Geometry: final body of the model. Coordinates: model frame, mm. A direction names the side the tool comes from. Give positions to 0.01 mm unless a question says otherwise; leave off trailing zeros. Order: outer loops, then holes, each group sorted by start corner. A loop starts at its lowest first (then second) coordinate and runs counter-clockwise, first axis right, second up. Notation, with made-up numbers: (-24.5, 85) - (-20.5, 85) arc R27 ccw to (-20.5, 101) - close; hole circle Ø5 at (87.25, 37.25). An arc over 180 degrees is marked (long way). One line per item, written item: value.
```python
from build123d import *

# Parameters (mm, degrees)
SKETCH_1_R          = 12.5
EXTRUDE_1_DEPTH     = 8.2
SKETCH_2_R          = 12.5
EXTRUDE_2_DEPTH     = 3
SKETCH_3_W          = 10
SKETCH_3_H          = 10
EXTRUDE_3_DEPTH     = 11.2
FILLET_1_R          = 10
SKETCH_4_R          = 2.5
CUT_EXTRUDE_4_DEPTH = 28.240939498
SKETCH_5_R          = 5.5
CUT_EXTRUDE_5_DEPTH = 4


with BuildPart() as part:
    # Эскиз1 → Вытянуть1 (new body)
    with BuildSketch(Plane(origin=(0, 0, 0), x_dir=(1, 0, 0), z_dir=(0, 1, 0))):
        with Locations(Location((0, 0, 0), (0, 0, 270))):
            Circle(SKETCH_1_R)
        Polygon((8.5, -4.907477288), (8.5, 4.907477288), (0, 9.814954576), (-8.5, 4.907477288), (-8.5, -4.907477288), (0, -9.814954576), align=None, mode=Mode.SUBTRACT)
    extrude(amount=EXTRUDE_1_DEPTH)

    # Эскиз2 → Вытянуть2 (add)
    with BuildSketch(Plane(origin=(0, 8.2, 0), x_dir=(1, 0, 0), z_dir=(0, 1, 0))):
        with Locations(Location((0, 0, 0), (0, 0, 270))):
            Circle(SKETCH_2_R)
    extrude(amount=EXTRUDE_2_DEPTH)

    # Эскиз3 → Вытянуть3 (add)
    with BuildSketch(Plane.XZ):
        with Locations((16.456439237, 0)):
            Rectangle(SKETCH_3_W, SKETCH_3_H)
        with Locations((-16.456439237, 0)):
            Rectangle(SKETCH_3_W, SKETCH_3_H)
    extrude(amount=-EXTRUDE_3_DEPTH)

    # Скругление1
    fillet_1_edges = [part.edges().sort_by_distance(p)[0] for p in [
        (11.456439237, 5.6, 5),
        (11.456439237, 5.6, -5),
        (-11.456439237, 5.6, -5),
        (-11.456439237, 5.6, 5),
    ]]
    fillet(fillet_1_edges, radius=FILLET_1_R)

    # Эскиз4 → Вытянуть4 (cut, through all)
    with BuildSketch(Plane(origin=(0, 11.2, 0), x_dir=(1, 0, 0), z_dir=(0, 1, 0))):
        with Locations(Location((16.456439237, 0, 0), (0, 0, 270))):
            Circle(SKETCH_4_R)
        with Locations(Location((-16.456439237, 0, 0), (0, 0, 270))):
            Circle(SKETCH_4_R)
    extrude(amount=-CUT_EXTRUDE_4_DEPTH, mode=Mode.SUBTRACT)

    # Эскиз5 → Вытянуть5 (cut)
    with BuildSketch(Plane(origin=(0, 11.2, 0), x_dir=(1, 0, 0), z_dir=(0, 1, 0))):
        with Locations(Location((0, 0, 0), (0, 0, 270))):
            Circle(SKETCH_5_R)
    extrude(amount=-CUT_EXTRUDE_5_DEPTH, mode=Mode.SUBTRACT)


solid = part.part
```
1) Section B-B, the plane x = 17.5. Return loops of the section in (y, z).
Answers below:
outline: (0, -5) - (11.2, -5) - (11.2, -2.27) - (0, -2.27) - close; (0, 2.27) - (11.2, 2.27) - (11.2, 5) - (0, 5) - close
2) Material intervals for line 1 along X through (y, z) = (10.5, 0); line 2 along X through (y, z) = (3.25, 0); line 3 along X through (y, z) = (1, 3), sorted ascending.
Answers below:
line 1: -21.46 to -18.96, -13.96 to -5.5, 5.5 to 13.96, 18.96 to 21.46
line 2: -21.46 to -18.96, -13.96 to -8.5, 8.5 to 13.96, 18.96 to 21.46
line 3: -21.46 to -8.5, 8.5 to 21.46
3) Section D-D, the plane z = 7.5. Return loops of the section in (x, y).
Answers below:
outline: (-10.16, 0) - (-4.01, 0) - (-4.01, 8.2) - (4.01, 8.2) - (4.01, 0) - (10.16, 0) - (10.16, 11.2) - (-10.16, 11.2) - close
4) Section A-A, the plane z = 0. Return loops of the section in (x, y).
Answers below:
outline: (-21.46, 0) - (-18.96, 0) - (-18.96, 11.2) - (-21.46, 11.2) - close; (-13.96, 0) - (-8.5, 0) - (-8.5, 8.2) - (-5.5, 8.2) - (-5.5, 11.2) - (-13.96, 11.2) - close; (5.5, 8.2) - (8.5, 8.2) - (8.5, 0) - (13.96, 0) - (13.96, 11.2) - (5.5, 11.2) - close; (18.96, 0) - (21.46, 0) - (21.46, 11.2) - (18.96, 11.2) - close
5) Set-up query: faces 1 (the face through (-19, 6, -5)), 2 (the face through (-19, 6, 5)), 3 (the face through (-4.191, 4.043, -7.396)). Return all of +Z, -Z, +X, -X, +Y, -Y with unobstructed straight access to the full face (end or side cutting, diameter ignored); none if empty.
Answers below:
face 1: -Z, -X, +Y, -Y
face 2: +Z, -X, +Y, -Y
face 3: -Y
6) Mould query, pull axis Z, two halves, no side actions, for faces 4 (the face through (12.634, 5.678, -5.895)), 5 (the face through (8.5, 4, 0)), 6 (the face through (-4, 0, 8)), 7 (the face through (-8.5, 4, 0)). Classes: released by +Z, released by -Z, zero draft, split by the parting line, or undercut.
Answers below:
face 4: released by -Z
face 5: undercut
face 6: zero draft
face 7: undercut
7) Section C-C, the plane y = 10. Return loops of the section in (x, z), then the cut area to 3 significant figures.
Answers below:
outline: (-21.46, -5) - (-16.77, -5) arc R10 cw to (-9.32, -8.33) arc R12.5 ccw to (9.32, -8.33) arc R10 cw to (16.77, -5) - (21.46, -5) - (21.46, 5) - (16.77, 5) arc R10 cw to (9.32, 8.33) arc R12.5 ccw to (-9.32, 8.33) arc R10 cw to (-16.77, 5) - (-21.46, 5) - close; hole circle Ø5 at (-16.46, 0); hole circle Ø11 at (0, 0); hole circle Ø5 at (16.46, 0)
area: 557 mm^2
8) First-contact query: pin 1 (3.5 mm diameter, centred on x = -18.5, y = 7, fed in from +Z); pin 2 (1 mm diameter, centred on x = -11, y = 7, fed in from +Z); pin 3 (8.5 mm diameter, centred on x = 2, z = 1, fed in from -Y); pin 4 (4.5 mm diameter, centred on x = -16.46, z = 0, fed in from +Y). Flat tips, straight axial feed; report the tip coordinate or a pass-through.
Answers below:
pin 1: z = 5
pin 2: z = 7.21
pin 3: y = 8.2
pin 4: through
